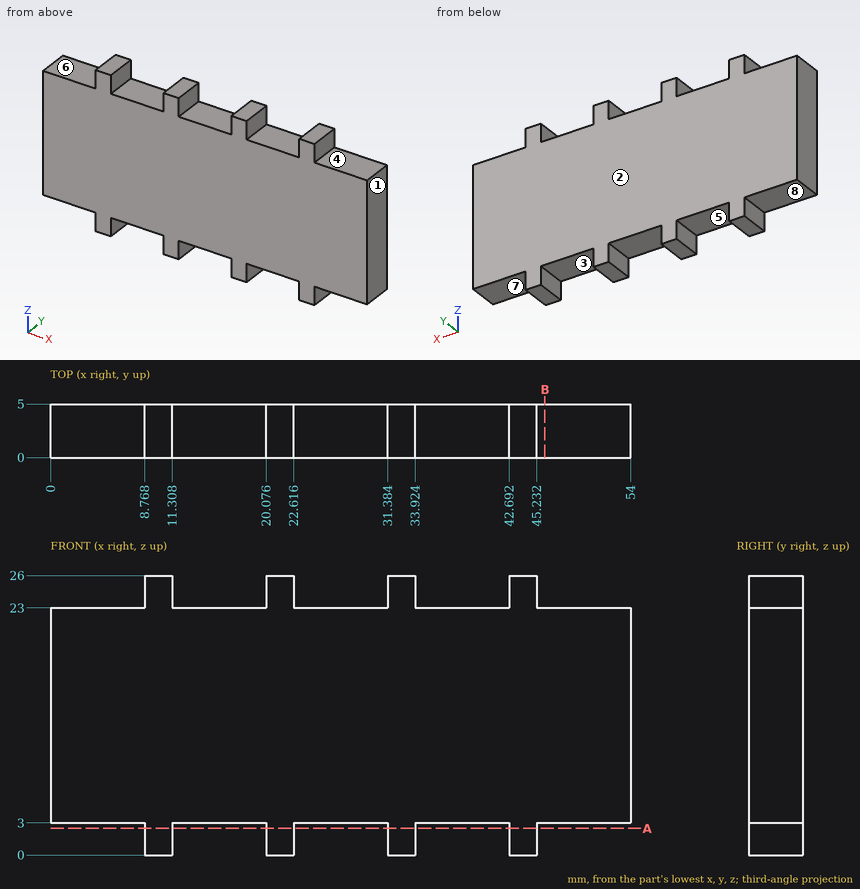
The drawing under review shows one solid part. Ordinate dimensions are in mm from its lowest x, y, z. A direction names the side the tool comes from. Coordinates: 2 decimals unless noted, no trailing zeros. Order: outer loops, then holes, each group sorted by start corner. A loop starts at its lowest first (then second) coordinate and runs counter-clockwise, first axis right, second up. Notation, with made-up numbers: M -28,74.25 L -17,74.25 A8 cw -17,84.25 Z; hole C -2,29.25 d2. An arc over 180 degrees is marked long. One line per question, with ' | ' between items.
(1) Add section A-A, the plane z = 2.5. Write out the cut boundary in (x, y), then the cut area to 3 significant figures.
Geometry results:
outline: M 8.77,0 L 11.31,0 L 11.31,5 L 8.77,5 Z; M 20.08,0 L 22.62,0 L 22.62,5 L 20.08,5 Z; M 31.38,0 L 33.92,0 L 33.92,5 L 31.38,5 Z; M 42.69,0 L 45.23,0 L 45.23,5 L 42.69,5 Z | area: 50.8 mm²
(2) Insertion check: pin 1 (2.5 mm diameter, centred on y = 2.5, z = 24.5, fed in from -X); pin 2 (0.9 mm diameter, centred on y = 2.5, z = 25, fed in from +X); pin 3 (1.5 mm diameter, centred on x = 50.5, y = 1.5, fed in from -Z). Each pin has a flat end and moves straight along its axis. Give the tip position at first contact, or say it passes through.
Geometry results:
pin 1: stops at x = 8.77 | pin 2: stops at x = 45.23 | pin 3: stops at z = 3
(3) For probe 1 along Z at (x, y) = (12.5, 1.25), list the stretches that pass through material, from the lowest coordinate up. Write a range as from..to.
Geometry results:
probe 1: z = 3..23
(4) Machinability: for the marked faces 4, 5, 6, 7 and 8, which of the approach directions +Z, -Z, +X, -X, +Y, -Y give a long, thin tool a straight path to every point of the face, cutting with its end or side? Answer none if there is none.
Geometry results:
face 4: +Z, +X, +Y, -Y | face 5: -Z, +Y, -Y | face 6: +Z, -X, +Y, -Y | face 7: -Z, +X, +Y, -Y | face 8: -Z, -X, +Y, -Y
(5) Add section B-B, the plane x = 46. Write out the cut boundary in (y, z), then the cut area to 3 significant figures.
Geometry results:
outline: M 0,3 L 5,3 L 5,23 L 0,23 Z | area: 100 mm²
(6) The part is to be moulded in two halves that separate along X. For the marked faces 1, 2 and 3, say which applies: +X half, -X half, draft (parallel to the pull), parting line (faces both ways), or undercut.
Geometry results:
face 1: +X half | face 2: draft | face 3: undercut
